```python
from build123d import *
from OCP.BRepFilletAPI import BRepFilletAPI_MakeChamfer

# Parameters (mm, degrees)
SKETCH1_W                      = 30
SKETCH1_H                      = 40
SKETCH1_R                      = 9.525
BOSS_EXTRUDE1_DEPTH            = 15
CHAMFER2_SIZE                  = 0.5
CHAMFER2_SIZE2                 = 0.866025404
CHAMFER3_SIZE                  = 0.5
M3X0_5_TAPPED_HOLE1_AT_2_COUNT = 2
M3X0_5_TAPPED_HOLE1_AT_2_PITCH = 20
M3X0_5_TAPPED_HOLE1_AT_3_COUNT = 2
M3X0_5_TAPPED_HOLE1_AT_3_PITCH = 10
M3X0_5_TAPPED_HOLE1_AT_4_COUNT = 2
M3X0_5_TAPPED_HOLE1_AT_4_PITCH = 10
M3X0_5_TAPPED_HOLE1_AT_5_COUNT = 2
M3X0_5_TAPPED_HOLE1_AT_5_PITCH = 10
M3X0_5_TAPPED_HOLE1_AT_6_COUNT = 2
M3X0_5_TAPPED_HOLE1_AT_6_PITCH = 22.360679775
M3X0_5_TAPPED_HOLE1_AT_7_COUNT = 2
M3X0_5_TAPPED_HOLE1_AT_7_PITCH = 22.360679775
M3X0_5_TAPPED_HOLE1_AT_8_COUNT = 2
M3X0_5_TAPPED_HOLE1_AT_8_PITCH = 14.142135624
M3X0_5_TAPPED_HOLE1_AT_9_COUNT = 2
M3X0_5_TAPPED_HOLE1_AT_9_PITCH = 14.142135624
CIRPATTERN1_COUNT              = 2


with BuildPart() as part:
    # Sketch1 → Boss-Extrude1 (new, symmetric)
    with BuildSketch(Plane.XY):
        Rectangle(SKETCH1_W, SKETCH1_H)
        Circle(SKETCH1_R, mode=Mode.SUBTRACT)
    extrude(amount=BOSS_EXTRUDE1_DEPTH, both=True)

    # Chamfer2: one chamfer whose edges measure the first distance from different faces: ONE call of the kernel's chamfer builder (chamfer() names one face for all edges)
    chamfer2_edges_1 = [part.edges().sort_by_distance(p)[0] for p in [
        (-9.525, 0, -15),
    ]]
    chamfer2_side_1 = [part.faces().sort_by_distance(p)[0] for p in [
        (0, -19.5, -15),
    ]]
    chamfer2_edges_2 = [part.edges().sort_by_distance(p)[0] for p in [
        (-9.525, 0, 15),
    ]]
    chamfer2_side_2 = [part.faces().sort_by_distance(p)[0] for p in [
        (-9.525, 0, 0),
    ]]
    chamfer2 = BRepFilletAPI_MakeChamfer(part.part.solid().wrapped)
    for e in chamfer2_edges_1:
        chamfer2.Add(CHAMFER2_SIZE, CHAMFER2_SIZE2, e.wrapped, chamfer2_side_1[0].wrapped)  # the first distance lies on this face
    for e in chamfer2_edges_2:
        chamfer2.Add(CHAMFER2_SIZE, CHAMFER2_SIZE2, e.wrapped, chamfer2_side_2[0].wrapped)  # the first distance lies on this face
    add(Compound.cast(chamfer2.Shape()), mode=Mode.REPLACE)

    # Chamfer3
    chamfer3_edges = [part.edges().sort_by_distance(p)[0] for p in [
        (0, 20, -15),
        (0, -20, -15),
    ]]
    chamfer(chamfer3_edges, length=CHAMFER3_SIZE)

    # Sketch8 → M3x0.5 Tapped Hole1 (revolve, cut)
    with BuildSketch(Plane(origin=(-10, 20, 0), x_dir=(0, 0, 1), z_dir=(1, 0, 0))):
        Polygon((0, 0), (0, 12.751075774), (1.25, 12), (1.25, 0), align=None)
    m3x0_5_tapped_hole1 = revolve(axis=Axis((-10, 26.35, 0), (0, -1, 0)), mode=Mode.SUBTRACT)

    # M3x0.5 Tapped Hole1 at 2: M3x0.5 Tapped Hole1 ×2
    with Locations(*[(i * M3X0_5_TAPPED_HOLE1_AT_2_PITCH, 0, 0) for i in range(1, M3X0_5_TAPPED_HOLE1_AT_2_COUNT)]):
        add(m3x0_5_tapped_hole1, mode=Mode.SUBTRACT)

    # M3x0.5 Tapped Hole1 at 3: M3x0.5 Tapped Hole1 ×2
    with Locations(*[(i * M3X0_5_TAPPED_HOLE1_AT_3_PITCH, 0, 0) for i in range(1, M3X0_5_TAPPED_HOLE1_AT_3_COUNT)]):
        add(m3x0_5_tapped_hole1, mode=Mode.SUBTRACT)

    # M3x0.5 Tapped Hole1 at 4: M3x0.5 Tapped Hole1 ×2
    with Locations(*[(0, 0, -i * M3X0_5_TAPPED_HOLE1_AT_4_PITCH) for i in range(1, M3X0_5_TAPPED_HOLE1_AT_4_COUNT)]):
        add(m3x0_5_tapped_hole1, mode=Mode.SUBTRACT)

    # M3x0.5 Tapped Hole1 at 5: M3x0.5 Tapped Hole1 ×2
    with Locations(*[(0, 0, i * M3X0_5_TAPPED_HOLE1_AT_5_PITCH) for i in range(1, M3X0_5_TAPPED_HOLE1_AT_5_COUNT)]):
        add(m3x0_5_tapped_hole1, mode=Mode.SUBTRACT)

    # M3x0.5 Tapped Hole1 at 6: M3x0.5 Tapped Hole1 ×2
    with Locations(*[Vector(0.894427190999916, 0, -0.44721359549995787) * (i * M3X0_5_TAPPED_HOLE1_AT_6_PITCH) for i in range(1, M3X0_5_TAPPED_HOLE1_AT_6_COUNT)]):
        add(m3x0_5_tapped_hole1, mode=Mode.SUBTRACT)

    # M3x0.5 Tapped Hole1 at 7: M3x0.5 Tapped Hole1 ×2
    with Locations(*[Vector(0.8944271909999159, 0, 0.447213595499958) * (i * M3X0_5_TAPPED_HOLE1_AT_7_PITCH) for i in range(1, M3X0_5_TAPPED_HOLE1_AT_7_COUNT)]):
        add(m3x0_5_tapped_hole1, mode=Mode.SUBTRACT)

    # M3x0.5 Tapped Hole1 at 8: M3x0.5 Tapped Hole1 ×2
    with Locations(*[Vector(0.7071067811865476, 0, -0.7071067811865475) * (i * M3X0_5_TAPPED_HOLE1_AT_8_PITCH) for i in range(1, M3X0_5_TAPPED_HOLE1_AT_8_COUNT)]):
        add(m3x0_5_tapped_hole1, mode=Mode.SUBTRACT)

    # M3x0.5 Tapped Hole1 at 9: M3x0.5 Tapped Hole1 ×2
    with Locations(*[Vector(0.7071067811865475, 0, 0.7071067811865476) * (i * M3X0_5_TAPPED_HOLE1_AT_9_PITCH) for i in range(1, M3X0_5_TAPPED_HOLE1_AT_9_COUNT)]):
        add(m3x0_5_tapped_hole1, mode=Mode.SUBTRACT)

    # CirPattern1: M3x0.5 Tapped Hole1 ×2 about axis
    cirpattern1_axis = Axis((0, 0, 15), (0, 0, -1))
    for i in range(1, CIRPATTERN1_COUNT):
        add(m3x0_5_tapped_hole1.rotate(cirpattern1_axis, i * 360 / CIRPATTERN1_COUNT), mode=Mode.SUBTRACT)

    # CirPattern1 copy 1 sketch → CirPattern1 copy 1 (revolve, cut)
    with BuildSketch(Plane(origin=(-10, -20, 0), x_dir=(0, 0, 1), z_dir=(-1, 0, 0))):
        Polygon((0, 0), (0, 12.751075774), (1.25, 12), (1.25, 0), align=None)
    revolve(axis=Axis((-10, -26.35, 0), (0, 1, 0)), mode=Mode.SUBTRACT)

    # CirPattern1 copy 2 sketch → CirPattern1 copy 2 (revolve, cut)
    with BuildSketch(Plane(origin=(0, -20, 0), x_dir=(0, 0, 1), z_dir=(-1, 0, 0))):
        Polygon((0, 0), (0, 12.751075774), (1.25, 12), (1.25, 0), align=None)
    revolve(axis=Axis((0, -26.35, 0), (0, 1, 0)), mode=Mode.SUBTRACT)

    # CirPattern1 copy 3 sketch → CirPattern1 copy 3 (revolve, cut)
    with BuildSketch(Plane(origin=(10, -20, -10), x_dir=(0, 0, 1), z_dir=(-1, 0, 0))):
        Polygon((0, 0), (0, 12.751075774), (1.25, 12), (1.25, 0), align=None)
    revolve(axis=Axis((10, -26.35, -10), (0, 1, 0)), mode=Mode.SUBTRACT)

    # CirPattern1 copy 4 sketch → CirPattern1 copy 4 (revolve, cut)
    with BuildSketch(Plane(origin=(10, -20, 10), x_dir=(0, 0, 1), z_dir=(-1, 0, 0))):
        Polygon((0, 0), (0, 12.751075774), (1.25, 12), (1.25, 0), align=None)
    revolve(axis=Axis((10, -26.35, 10), (0, 1, 0)), mode=Mode.SUBTRACT)

    # CirPattern1 copy 5 sketch → CirPattern1 copy 5 (revolve, cut)
    with BuildSketch(Plane(origin=(-10, -20, -10), x_dir=(0, 0, 1), z_dir=(-1, 0, 0))):
        Polygon((0, 0), (0, 12.751075774), (1.25, 12), (1.25, 0), align=None)
    revolve(axis=Axis((-10, -26.35, -10), (0, 1, 0)), mode=Mode.SUBTRACT)

    # CirPattern1 copy 6 sketch → CirPattern1 copy 6 (revolve, cut)
    with BuildSketch(Plane(origin=(-10, -20, 10), x_dir=(0, 0, 1), z_dir=(-1, 0, 0))):
        Polygon((0, 0), (0, 12.751075774), (1.25, 12), (1.25, 0), align=None)
    revolve(axis=Axis((-10, -26.35, 10), (0, 1, 0)), mode=Mode.SUBTRACT)

    # CirPattern1 copy 7 sketch → CirPattern1 copy 7 (revolve, cut)
    with BuildSketch(Plane(origin=(0, -20, -10), x_dir=(0, 0, 1), z_dir=(-1, 0, 0))):
        Polygon((0, 0), (0, 12.751075774), (1.25, 12), (1.25, 0), align=None)
    revolve(axis=Axis((0, -26.35, -10), (0, 1, 0)), mode=Mode.SUBTRACT)

    # CirPattern1 copy 8 sketch → CirPattern1 copy 8 (revolve, cut)
    with BuildSketch(Plane(origin=(0, -20, 10), x_dir=(0, 0, 1), z_dir=(-1, 0, 0))):
        Polygon((0, 0), (0, 12.751075774), (1.25, 12), (1.25, 0), align=None)
    revolve(axis=Axis((0, -26.35, 10), (0, 1, 0)), mode=Mode.SUBTRACT)

    # Chamfer6
    # the kernel refuses this chamfer: 0.5 mm, written as the material it takes off along each edge
    with BuildSketch(Plane(origin=(14.666666667, -19.666666667, 14.666666667), x_dir=(0.7071067811865475, 0.7071067811865475, 0), z_dir=(0.5773502691896258, -0.5773502691896258, 0.5773502691896258)), Plane(origin=(-14.666666667, -19.666666667, 14.666666667), x_dir=(0, 0.7071067811865475, 0.7071067811865475), z_dir=(-0.5773502691896258, -0.5773502691896258, 0.5773502691896258))) as chamfer6_piece_1:
        Polygon((-0.353553391, -0.204124145), (0.353553391, -0.204124145), (0, 0.40824829), align=None)
    extrude(amount=0.635085296, mode=Mode.SUBTRACT)
    with BuildSketch(Plane(origin=(14.666666667, 19.666666667, 14.666666667), x_dir=(-0.7071067811865475, 0, 0.7071067811865475), z_dir=(0.5773502691896258, 0.5773502691896258, 0.5773502691896258)), Plane(origin=(-14.666666667, 19.666666667, 14.666666667), x_dir=(-0.7071067811865475, 0, -0.7071067811865475), z_dir=(-0.5773502691896258, 0.5773502691896258, 0.5773502691896258))) as chamfer6_piece_2:
        Polygon((-0.353553391, 0.204124145), (0.353553391, 0.204124145), (0, -0.40824829), align=None)
    extrude(amount=0.635085296, mode=Mode.SUBTRACT)
    with BuildSketch(Plane(origin=(15, -20.785841494, -15), x_dir=(0.027495876610585647, 0, 0.9996219169112968), z_dir=(0, 1, 0)), Plane(origin=(-15, 20.785841494, -15), x_dir=(-0.027495876610585647, 0, 0.9996219169112968), z_dir=(0, -1, 0))) as chamfer6_piece_3:
        with BuildLine():
            Line((0.514336598, 0), (-0.028273577, -0.513558897))
            Line((-0.028273577, -0.513558897), (-0.038269797, -0.513283938))
            ThreePointArc((-0.038269797, -0.513283938), (-0.017064614, -0.256698915), (-0.009996219, 0.000274959))
            Line((-0.009996219, 0.000274959), (0.000274959, 0.009996219))
            ThreePointArc((0.000274959, 0.009996219), (0.257248832, 0.002927825), (0.514611556, 0.009996219))
            Line((0.514611556, 0.009996219), (0.514336598, 0))
        make_face()
    extrude(amount=41.571682988, mode=Mode.SUBTRACT)
    with BuildSketch(Plane(origin=(15, -21.285841494, 15), x_dir=(0.027495876610585647, 0, -0.9996219169112968), z_dir=(0, 1, 0))) as chamfer6_piece_4:
        with BuildLine():
            Line((0.514336598, 0), (-0.028273577, 0.513558897))
            Line((-0.028273577, 0.513558897), (-0.038269797, 0.513283938))
            ThreePointArc((-0.038269797, 0.513283938), (-0.017064614, 0.256698915), (-0.009996219, -0.000274959))
            Line((-0.009996219, -0.000274959), (0.000274959, -0.009996219))
            ThreePointArc((0.000274959, -0.009996219), (0.257248832, -0.002927825), (0.514611556, -0.009996219))
            Line((0.514611556, -0.009996219), (0.514336598, 0))
        make_face()
    extrude(amount=42.571682988, mode=Mode.SUBTRACT)
    with BuildSketch(Plane(origin=(15, 20, -15.785841494), x_dir=(0.02749587661058555, -0.9996219169112968, 0), z_dir=(0, 0, 1)), Plane(origin=(-15, 20, 16.285841494), x_dir=(-0.02749587661058555, -0.9996219169112968, 0), z_dir=(0, 0, -1)), Plane(origin=(-15, -20, 16.285841494), x_dir=(0.9996219169112968, -0.0274958766105891, 0), z_dir=(0, 0, -1)), Plane(origin=(15, -20, -15.785841494), x_dir=(-0.9996219169112968, -0.0274958766105891, 0), z_dir=(0, 0, 1))) as chamfer6_piece_5:
        with BuildLine():
            Line((0.514336598, 0), (-0.028273577, -0.513558897))
            Line((-0.028273577, -0.513558897), (-0.038269797, -0.513283938))
            ThreePointArc((-0.038269797, -0.513283938), (-0.017064614, -0.256698915), (-0.009996219, 0.000274959))
            Line((-0.009996219, 0.000274959), (0.000274959, 0.009996219))
            ThreePointArc((0.000274959, 0.009996219), (0.257248832, 0.002927825), (0.514611556, 0.009996219))
            Line((0.514611556, 0.009996219), (0.514336598, 0))
        make_face()
    extrude(amount=32.071682988, mode=Mode.SUBTRACT)
    with BuildSketch(Plane(origin=(16.285841494, 20, 15), x_dir=(0, -0.9996219169112968, 0.02749587661058555), z_dir=(-1, 0, 0))) as chamfer6_piece_6:
        with BuildLine():
            Line((0.514336598, 0), (-0.028273577, -0.513558897))
            Line((-0.028273577, -0.513558897), (-0.038269797, -0.513283938))
            ThreePointArc((-0.038269797, -0.513283938), (-0.017064614, -0.256698915), (-0.009996219, 0.000274959))
            Line((-0.009996219, 0.000274959), (0.000274959, 0.009996219))
            ThreePointArc((0.000274959, 0.009996219), (0.257248832, 0.002927825), (0.514611556, 0.009996219))
            Line((0.514611556, 0.009996219), (0.514336598, 0))
        make_face()
    extrude(amount=32.571682988, mode=Mode.SUBTRACT)
    with BuildSketch(Plane(origin=(-16.285841494, -20, 15), x_dir=(0, -0.0274958766105891, -0.9996219169112968), z_dir=(1, 0, 0))) as chamfer6_piece_7:
        with BuildLine():
            Line((0.514336598, 0), (-0.028273577, 0.513558897))
            Line((-0.028273577, 0.513558897), (-0.038269797, 0.513283938))
            ThreePointArc((-0.038269797, 0.513283938), (-0.017064614, 0.256698915), (-0.009996219, -0.000274959))
            Line((-0.009996219, -0.000274959), (0.000274959, -0.009996219))
            ThreePointArc((0.000274959, -0.009996219), (0.257248832, -0.002927825), (0.514611556, -0.009996219))
            Line((0.514611556, -0.009996219), (0.514336598, 0))
        make_face()
    extrude(amount=32.571682988, mode=Mode.SUBTRACT)
    with BuildSketch(Plane(origin=(-15, 21.285841494, 15), x_dir=(0.9996219169112968, 0, 0.027495876610585647), z_dir=(0, -1, 0))) as chamfer6_piece_8:
        with BuildLine():
            Line((0.514336598, 0), (-0.028273577, -0.513558897))
            Line((-0.028273577, -0.513558897), (-0.038269797, -0.513283938))
            ThreePointArc((-0.038269797, -0.513283938), (-0.017064614, -0.256698915), (-0.009996219, 0.000274959))
            Line((-0.009996219, 0.000274959), (0.000274959, 0.009996219))
            ThreePointArc((0.000274959, 0.009996219), (0.257248832, 0.002927825), (0.514611556, 0.009996219))
            Line((0.514611556, 0.009996219), (0.514336598, 0))
        make_face()
    extrude(amount=42.571682988, mode=Mode.SUBTRACT)


solid = part.part
```
The listing builds one solid part. Answer for the finished solid, in the listing's coordinates (mm). A direction names the side the tool comes from. Give positions to 0.01 mm unless a question says otherwise; leave off trailing zeros. Order: outer loops, then holes, each group sorted by start corner. A loop starts at its lowest first (then second) coordinate and runs counter-clockwise, first axis right, second up. Notation, with made-up numbers: (16.25, 22.25) -> (52.25, 22.25) arc R21 ccw to (52.25, 35.25) -> close; hole circle Ø11 at (40.5, 8.25). An arc over 180 degrees is marked (long way). Answer as a JSON object with one key per item and string values. Group by question number.
Item 1: The part is cut by section B-B on y = 14.5. Give the number of separate pieces and of enclosed holes in the cut face, and give its area (3 significant figures).
Item 2: Consider L1, parallel to X at y = -16.5, z = 0; L2, parallel to X at y = 12.5, z = 9.5. Determine where each line is inside the solid, lowest interval first. Write a range as from..to.
Item 3: The part is cut by section A-A on y = 0. Write down the section's boundary in (x, z) (3 decimals), and give its area (3 significant figures).
Item 4: Flat-ended cylindrical pins translate along their axes: pin 1 (2 mm diameter, centred on x = 10, z = -10, fed in from +Y); pin 2 (2 mm diameter, centred on x = 0, z = 10, fed in from +Y); pin 3 (1.5 mm diameter, centred on x = -10, z = 0, fed in from -Y); pin 4 (2 mm diameter, centred on x = 10, z = 0, fed in from -Y). Find the tip coordinate at first contact, or state that the pin passes through.
Item 5: A tool of negligible diameter and unlimited length cuts with its end or side. For faces 1 (the cylindrical face through (-10.845, 14.084, 9.079)), 2 (the flat face through (15, 0, 0)), 3 (the cylindrical face through (-9.95, -14.08, 8.75)), from which of +Z, -Z, +X, -X, +Y, -Y can it reach the whole face along a straight path? Write none if from no direction.
Item 6: Determine the mould class of faces 4 (the conical face through (10.08, 7.38, 0.2)), 5 (the conical face through (-10.08, -7.38, 0.2)), 6 (the cylindrical face through (-2.06, -9.3, -0.02)), 7 (the cylindrical face through (-8.946, -14.084, 0.672)) for opening direction Y: pulls with the +Y half, pulls with the -Y half, needs draft (parallel to the pull), parting line crosses it, or undercut.
Item 7: The part is cut by section C-C on z = 3.5. Write down the section's boundary in (x, y) (3 decimals), and give its area (3 significant figures).
Result set:
{
 "1": {"separate pieces": "1", "enclosed holes": "9", "area": "855 mm²"},
 "2": {"L1": "-15..-11.25, -8.75..-1.25, 1.25..8.75, 11.25..15", "L2": "-15..-11.15, -8.85..-1.15, 1.15..8.85, 11.15..15"},
 "3": {"outline": "(-15, -14.5) -> (-14.5, -15) -> (-10.025, -15) -> (-9.525, -14.134) -> (-9.525, 14.5) -> (-10.391, 15) -> (-14.5, 15) -> (-15, 14.5) -> close; (9.525, -14.134) -> (10.025, -15) -> (14.5, -15) -> (15, -14.5) -> (15, 14.5) -> (14.5, 15) -> (10.391, 15) -> (9.525, 14.5) -> close", "area": "327 mm²"},
 "4": {"pin 1": "y = 7.85", "pin 2": "through", "pin 3": "y = -7.7", "pin 4": "y = -7.85"},
 "5": {"face 1": "+Y", "face 2": "+Z, -Z, +X, +Y, -Y", "face 3": "-Y"},
 "6": {"face 4": "pulls with the +Y half", "face 5": "pulls with the -Y half", "face 6": "undercut", "face 7": "needs draft"},
 "7": {"outline": "(-15, -19.5) -> (-14.5, -20) -> (14.5, -20) -> (15, -19.5) -> (15, 19.5) -> (14.5, 20) -> (-14.5, 20) -> (-15, 19.5) -> close; hole circle Ø19.05 at (0, 0)", "area": "914 mm²"}
}
